Autodesk Inventor part; units mm, degrees
ref_plane "Work Plane1" through (0, 5, 0) normal (0, 1, 0) x (1, 0, 0)
ref_plane "Work Plane2" through (0, 10, 0) normal (0, 1, 0) x (1, 0, 0)
ref_plane "Work Plane3" through (0, 10, 0) normal (0, 1, 0) x (1, 0, 0)
ref_plane "Work Plane1" through (0, 5, 0) normal (0, 1, 0) x (1, 0, 0)
sketch "Sketch2" plane through (0, 5, 0) normal (0, 1, 0) x (1, 0, 0)
  line L0 (0, 0) -> (0, 60)
  line L1 (0, 60) -> (-17.2323, 107.3454)
  line L2 (10, 0) -> (-10, 0)
  line L3 (-10, 0) -> (-10, 60)
  line L4 (-10, 60) -> (10, 60)
  line L5 (10, 60) -> (10, 0)
  line L6 (10, 0) -> (-10, 60) construction
  line L7 (-10, 0) -> (10, 60) construction
  line L8 (-17.2323, 107.3454) -> (-7.8354, 110.7656)
  line L9 (-7.8354, 110.7656) -> (10, 60)
  line L10 (0, 60) -> (-9.3969, 56.5798)
  line L11 (-9.3969, 56.5798) -> (-26.0986, 104.1184)
  line L12 (-26.0986, 104.1184) -> (-17.2323, 107.3454)
  point P0 (0, 30)
  dimension "d3" = 60
  dimension "d4" = 160
  dimension "d5" = 20
  dimension "d6" = 60
  dimension "d9" = 10
  dimension "d10" = 10
extrude "Extrusion2" add sketch "Sketch2" along normal blind 5 contours L2 L3 L11 L10 L0 | L0 L4 L5 L2 | L4 L3 L11 L12 L1 | L10 L11 L3 L4
ref_plane "Work Plane2" through (0, 10, 0) normal (0, 1, 0) x (1, 0, 0)
sketch "Sketch3" plane through (0, 10, 0) normal (0, 1, 0) x (1, 0, 0)
  line L0 (0, 60) -> (-17.2323, 107.3454)
  line L1 (-17.2323, 107.3454) -> (-26.0986, 104.1184)
  line L2 (-17.2323, 107.3454) -> (-7.7976, 110.66)
  line L3 (10, 60) -> (0, 60)
  line L4 (-7.7976, 110.66) -> (10, 60)
  line L5 (0, 60) -> (-17.2323, 107.3454)
  line L6 (10, 60) -> (0, 60)
  line L7 (0, 60) -> (-17.2323, 107.3454)
  point P0 (0, 0)
  dimension "d13" = 10
extrude "Extrusion3" add sketch "Sketch3" against normal blind 5
ref_plane "Work Plane3" through (0, 10, 0) normal (0, 1, 0) x (1, 0, 0)
sketch "Sketch4" plane through (0, 10, 0) normal (0, 1, 0) x (1, 0, 0)
  circle A0 centre (0, 0) radius 20
extrude "Extrusion4" add sketch "Sketch4" along normal blind 5
properties part number "scale_l_arm"
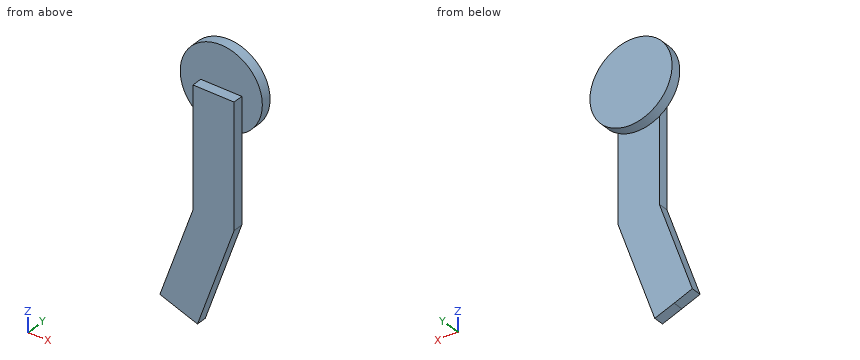
Source: CAD feature listing. Evaluate the final solid. Frame: model axes, mm. Coordinates: 2 decimals unless noted, no trailing zeros. Loops run counter-clockwise (first coordinate to the right, second up) from the corner with the lowest first, then second, coordinate; pieces in that order, holes last. Notation, with made-up numbers: (79, 35.5) - (116, 35.5) arc R28 cw to (116, 57.5) - close; hole circle Ø8 at (-24.75, 20.5). An arc over 180 degrees is marked (long way). One line per question, with ' | ' between items.
1) Section A-A, the plane y = 7.75. Return loops of the section in (x, z).
Report:
outline: (-26.1, -104.12) - (-17.23, -107.35) - (-7.8, -110.66) - (10, -60) - (10, 0) - (-10, 0) - (-10, -58.3) - close
2) Section C-C, the plane z = -38. Return loops of the section in (x, y), then the cut area to 3 significant figures.
Report:
outline: (-10, 5) - (10, 5) - (10, 10) - (-10, 10) - close | area: 100 mm²
3) Section B-B, the plane x = -6. Return loops of the section in (y, z).
Report:
outline: (5, -105.54) - (10, -105.54) - (10, -19.08) - (15, -19.08) - (15, 19.08) - (10, 19.08) - (10, 0) - (5, 0) - close
4) Section D-D, the plane x = 0. Return loops of the section in (y, z), then the cut area to 3 significant figures.
Report:
outline: (5, -88.46) - (10, -88.46) - (10, -20) - (15, -20) - (15, 20) - (10, 20) - (10, 0) - (5, 0) - close | area: 642 mm²
5) Line query: line 1 along Y through (x, z) = (-5, 6); line 2 along X through (y, z) = (14, -1); line 3 along X through (y, z) = (5.75, -40.5). Output: solid intervals per line, ascending.
Report:
line 1: y = 10 to 15 | line 2: x = -19.97 to 19.97 | line 3: x = -10 to 10
6) First-contact query: P1, Ø5, axis at x = -5, y = 11.5, coming from the +Z side; P2, Ø2.5, axis at x = -0.5, y = 6.5, coming from the +Z side; P3, Ø1, axis at x = -9, y = 12, coming from the +Z side. Flat tips, straight axial feed; report the tip coordinate or a pass-through.
Report:
P1: stops at z = 19.84 | P2: stops at z = 0 | P3: stops at z = 18.1
